Check sheet for the modelled part. Datum: model origin and axes. Units: mm. A direction names the side the tool comes from. Round coordinates to 2 decimals unless told otherwise and drop trailing zeros. Order: outer loops, then holes, each group sorted by start corner. A loop starts at its lowest first (then second) coordinate and runs counter-clockwise, first axis right, second up.
(1) Sectioned sample at A-A, the plane y = -25.5. Enter the section's corners in (x, z).
(2) Sectioned sample at C-C, the plane y = -32. Enter the section's corners in (x, z).
(3) Tool access check on faces 5 (the flat face through (-20, -45.939, -3)), 6 (the flat face through (18, -48, -11.938)), 7 (the flat face through (-19, -45, 20.828)), 8 (the flat face through (20, -46.99, -15)), 9 (the flat face through (0, -9, -16.51)). Record the directions out of +Z, -Z, +X, -X, +Y, -Y that give a thin tool (end or side, any length) a straight path to the whole face; none if there is none.
(4) Sectioned sample at B-B, the plane y = -40. Enter the section's corners in (x, z), and give its area (3 significant figures).
(5) Depth check by flat-ended pin: pin 1 (12.5 mm diameter, centred on x = -5.5, y = -47, fed in from -Z); pin 2 (16 mm diameter, centred on y = -41.5, z = -7.5, fed in from -X); pin 3 (1.5 mm diameter, centred on y = -15, z = 4, fed in from +X). Enter the tip coordinate at first touch or a pass-through.
(6) Mould release check, pull along Z, two halves, no side actions. Record for faces 1 (the flat face through (-18, -45, -22.86)), 2 (the cylindrical face through (-10.05, -4.29, 13.1)), 3 (the flat face through (14.195, -60.53, -0.107)), 4 (the flat face through (19, -45, -20.828)): released by +Z, released by -Z, zero draft, split by the parting line, or undercut.
(7) Thickness scan on probe 1 along Y at (x, z) = (19, 5.5); probe 2 along Z at (x, y) = (20.5, -54); probe 3 along Y at (x, z) = (6, -13). Record the ranges inside material, lowest first.
```python
from build123d import *

# Parameters (mm, degrees)
SKETCH1_R           = 12.446
BOSS_EXTRUDE1_DEPTH = 1.524
SKETCH2_R           = 16.51
BOSS_EXTRUDE2_DEPTH = 5.08
BOSS_EXTRUDE3_DEPTH = 5.842
FILLET1_R           = 0.508
FILLET2_R           = 0.508
SKETCH4_R           = 13.97
BOSS_EXTRUDE4_DEPTH = 4.064
BOSS_EXTRUDE5_DEPTH = 10.414
SKETCH6_W           = 22.86
SKETCH6_H           = 40.64
BOSS_EXTRUDE6_DEPTH = 34.798
SKETCH7_R           = 2.286
CUT_EXTRUDE1_DEPTH  = 9.398
SKETCH9_W           = 45.72
SKETCH9_H           = 34.798
BOSS_EXTRUDE7_DEPTH = 12.7
SKETCH10_W          = 41.656
SKETCH10_H          = 34.798
CUT_EXTRUDE2_DEPTH  = 9.652
CUT_EXTRUDE4_DEPTH  = 81.511990312
CUT_EXTRUDE5_DEPTH  = 81.511990312
SKETCH13_W          = 6.858
SKETCH13_H          = 1.524
BOSS_EXTRUDE8_DEPTH = 7.112
SKETCH14_W          = 6.604
SKETCH14_H          = 1.524
BOSS_EXTRUDE9_DEPTH = 7.112
SKETCH16_R          = 1.524
CUT_EXTRUDE7_DEPTH  = 7.112
SKETCH17_R          = 1.524
CUT_EXTRUDE8_DEPTH  = 12.7
FILLET3_R           = 1.27


with BuildPart() as part:
    # Sketch1 → Boss-Extrude1 (new body)
    with BuildSketch(Plane(origin=(0, 0, 0), x_dir=(1, 0, 0), z_dir=(0, 1, 0))):
        with Locations(Location((0, 0, 0), (0, 0, 270))):
            Circle(SKETCH1_R)
    extrude(amount=-BOSS_EXTRUDE1_DEPTH)

    # Sketch2 → Boss-Extrude2 (add)
    with BuildSketch(Plane.XZ.offset(1.524)):
        with Locations(Location((0, 0, 0), (0, 0, 270))):
            Circle(SKETCH2_R)
    extrude(amount=BOSS_EXTRUDE2_DEPTH)

    # Sketch3 → Boss-Extrude3 (add)
    with BuildSketch(Plane.XZ.offset(6.604)):
        Polygon((16.51, 7.366), (16.51, -7.366), (7.366, -16.51), (-7.366, -16.51), (-16.51, -7.366), (-16.51, 7.366), (-7.366, 16.51), (7.366, 16.51), align=None)
    extrude(amount=BOSS_EXTRUDE3_DEPTH)

    # Fillet1
    fillet1_edges = [part.edges().sort_by_distance(p)[0] for p in [
        (0, -1.524, 16.51),
    ]]
    fillet(fillet1_edges, radius=FILLET1_R)

    # Fillet2
    fillet2_edges = [part.edges().sort_by_distance(p)[0] for p in [
        (7.366, -9.525, -16.51),
        (16.51, -9.525, -7.366),
        (16.51, -9.525, 7.366),
        (7.366, -9.525, 16.51),
        (-7.366, -9.525, 16.51),
        (-16.51, -9.525, 7.366),
        (-16.51, -9.525, -7.366),
        (-7.366, -9.525, -16.51),
    ]]
    fillet(fillet2_edges, radius=FILLET2_R)

    # Sketch4 → Boss-Extrude4 (add)
    with BuildSketch(Plane.XZ.offset(12.446)):
        with Locations(Location((0, 0, 0), (0, 0, 270))):
            Circle(SKETCH4_R)
    extrude(amount=BOSS_EXTRUDE4_DEPTH)

    # Sketch5 → Boss-Extrude5 (add)
    with BuildSketch(Plane.XZ.offset(16.51)):
        with BuildLine():
            Line((12.7, 20.32), (-12.7, 20.32))
            ThreePointArc((-12.7, 20.32), (-18.088153673, 18.088153673), (-20.32, 12.7))
            Line((-20.32, 12.7), (-20.32, -12.7))
            ThreePointArc((-20.32, -12.7), (-18.088153673, -18.088153673), (-12.7, -20.32))
            Line((-12.7, -20.32), (12.7, -20.32))
            ThreePointArc((12.7, -20.32), (18.088153673, -18.088153673), (20.32, -12.7))
            Line((20.32, -12.7), (20.32, 12.7))
            ThreePointArc((20.32, 12.7), (18.088153673, 18.088153673), (12.7, 20.32))
        make_face()
    extrude(amount=BOSS_EXTRUDE5_DEPTH)

    # Sketch6 → Boss-Extrude6 (add)
    with BuildSketch(Plane.XZ.offset(26.924)):
        Rectangle(SKETCH6_W, SKETCH6_H)
    extrude(amount=BOSS_EXTRUDE6_DEPTH)

    # Sketch7 → Cut-Extrude1 (cut)
    with BuildSketch(Plane.XZ.offset(61.722)):
        with Locations(Location((0, -12.7, 0), (0, 0, 270))):
            Circle(SKETCH7_R)
        with Locations(Location((0, 12.7, 0), (0, 0, 270))):
            Circle(SKETCH7_R)
    extrude(amount=-CUT_EXTRUDE1_DEPTH, mode=Mode.SUBTRACT)

    # Sketch9 → Boss-Extrude7 (add)
    with BuildSketch(Plane(origin=(11.43, 0, 0), x_dir=(0, 0, -1), z_dir=(1, 0, 0))):
        with Locations((0, -44.323)):
            Rectangle(SKETCH9_W, SKETCH9_H)
    boss_extrude7 = extrude(amount=BOSS_EXTRUDE7_DEPTH)

    # Mirror1: Boss-Extrude7 across plane
    add(boss_extrude7.mirror(Plane(origin=(0, 0, 0), x_dir=(0, 0, 1), z_dir=(1, 0, 0))))

    # Sketch10 → Cut-Extrude2 (cut)
    with BuildSketch(Plane(origin=(24.13, 0, 0), x_dir=(0, 0, -1), z_dir=(1, 0, 0))):
        with Locations((0, -44.323)):
            Rectangle(SKETCH10_W, SKETCH10_H)
    cut_extrude2 = extrude(amount=-CUT_EXTRUDE2_DEPTH, mode=Mode.SUBTRACT)

    # Mirror2: Cut-Extrude2 across plane
    add(cut_extrude2.mirror(Plane(origin=(0, 0, 0), x_dir=(0, 0, 1), z_dir=(1, 0, 0))), mode=Mode.SUBTRACT)

    # Sketch11 → Cut-Extrude4 (cut, through all)
    with BuildSketch(Plane(origin=(0, 0, -22.86), x_dir=(-1, 0, 0), z_dir=(0, 0, -1))):
        Polygon((-11.43, -26.924), (-24.13, -32.874707767), (-24.13, -26.924), align=None)
        Polygon((24.13, -32.874707767), (24.13, -26.924), (11.43, -26.924), align=None)
        Polygon((11.326658159, -61.931639732), (24.061569251, -56.056015305), (24.026436821, -62.006619362), align=None)
        Polygon((-24.197589663, -55.77109271), (-24.232722094, -61.721696766), (-11.532943432, -61.796676397), align=None)
    extrude(amount=-CUT_EXTRUDE4_DEPTH, mode=Mode.SUBTRACT)

    # Sketch12 → Cut-Extrude5 (cut, through all)
    with BuildSketch(Plane(origin=(0, 0, -22.86), x_dir=(-1, 0, 0), z_dir=(0, 0, -1))):
        Polygon((27.344093716, -61.722), (27.344093716, -56.075395365), (24.061569251, -56.056015305), (20.546985538, -61.722), align=None)
    extrude(amount=-CUT_EXTRUDE5_DEPTH, mode=Mode.SUBTRACT)

    # Sketch13 → Boss-Extrude8 (add)
    with BuildSketch(Plane(origin=(14.478, 0, 0), x_dir=(0, 0, -1), z_dir=(1, 0, 0))):
        with Locations((-3.429, -47.752)):
            Rectangle(SKETCH13_W, SKETCH13_H)
        with Locations((15.367, -47.752)):
            Rectangle(SKETCH13_W, SKETCH13_H)
    extrude(amount=BOSS_EXTRUDE8_DEPTH)

    # Sketch14 → Boss-Extrude9 (add)
    with BuildSketch(Plane.ZY.offset(14.478)):
        with Locations((-3.302, -45.176922844)):
            Rectangle(SKETCH14_W, SKETCH14_H)
        with Locations((16.764, -45.176922844)):
            Rectangle(SKETCH14_W, SKETCH14_H)
    extrude(amount=BOSS_EXTRUDE9_DEPTH)

    # Sketch16 → Cut-Extrude7 (cut)
    with BuildSketch(Plane.XZ.offset(45.938922844)):
        with Locations(Location((-18.034, -3.302, 0), (0, 0, 270))):
            Circle(SKETCH16_R)
        with Locations(Location((-18.034, 16.764, 0), (0, 0, 270))):
            Circle(SKETCH16_R)
        with Locations((18.034, 3.429)):
            Circle(SKETCH16_R)
        with Locations((18.034, -15.367)):
            Circle(SKETCH16_R)
    extrude(amount=-CUT_EXTRUDE7_DEPTH, mode=Mode.SUBTRACT)

    # Sketch17 → Cut-Extrude8 (cut)
    with BuildSketch(Plane(origin=(0, -38.1, 0), x_dir=(1, 0, 0), z_dir=(0, 1, 0))):
        with Locations(Location((18.034, 15.367, 0), (0, 0, 270))):
            Circle(SKETCH17_R)
        with Locations(Location((18.034, -3.429, 0), (0, 0, 270))):
            Circle(SKETCH17_R)
    extrude(amount=-CUT_EXTRUDE8_DEPTH, mode=Mode.SUBTRACT)

    # Fillet3
    fillet3_edges = [part.edges().sort_by_distance(p)[0] for p in [
        (-11.43, -44.323, -22.86),
        (11.43, -44.323, -22.86),
        (-11.43, -44.323, 22.86),
        (11.43, -44.323, 22.86),
    ]]
    fillet(fillet3_edges, radius=FILLET3_R)


solid = part.part
```
Derived:
1. outline: (-20.32, -12.7) arc R7.62 ccw to (-12.7, -20.32) - (12.7, -20.32) arc R7.62 ccw to (20.32, -12.7) - (20.32, 12.7) arc R7.62 ccw to (12.7, 20.32) - (-12.7, 20.32) arc R7.62 ccw to (-20.32, 12.7) - close
2. outline: (-22.26, -22.86) - (-12.7, -22.86) arc R1.27 ccw to (-11.43, -21.59) - (-11.43, -20.32) - (11.43, -20.32) - (11.43, -21.59) arc R1.27 ccw to (12.7, -22.86) - (22.26, -22.86) - (22.26, -20.83) - (14.48, -20.83) - (14.48, 20.83) - (22.26, 20.83) - (22.26, 22.86) - (12.7, 22.86) arc R1.27 ccw to (11.43, 21.59) - (11.43, 20.32) - (-11.43, 20.32) - (-11.43, 21.59) arc R1.27 ccw to (-12.7, 22.86) - (-22.26, 22.86) - (-22.26, 20.83) - (-14.48, 20.83) - (-14.48, -20.83) - (-22.26, -20.83) - close
3. face 5: -X, -Y
3. face 6: +X, -Y
3. face 7: -X, +Y, -Y
3. face 8: +X
3. face 9: -Z, +X, -X, +Y
4. outline: (-24.13, -22.86) - (-12.7, -22.86) arc R1.27 ccw to (-11.43, -21.59) - (-11.43, -20.32) - (11.43, -20.32) - (11.43, -21.59) arc R1.27 ccw to (12.7, -22.86) - (24.13, -22.86) - (24.13, -20.83) - (14.48, -20.83) - (14.48, 20.83) - (24.13, 20.83) - (24.13, 22.86) - (12.7, 22.86) arc R1.27 ccw to (11.43, 21.59) - (11.43, 20.32) - (-11.43, 20.32) - (-11.43, 21.59) arc R1.27 ccw to (-12.7, 22.86) - (-24.13, 22.86) - (-24.13, 20.83) - (-14.48, 20.83) - (-14.48, -20.83) - (-24.13, -20.83) - close
4. area: 1,280 mm2
5. pin 1: stops at z = -22.43
5. pin 2: stops at x = -21.59
5. pin 3: stops at x = 13.59
6. face 1: released by -Z
6. face 2: split by the parting line
6. face 3: zero draft
6. face 4: undercut
7. probe 1: y = -48.51 to -46.99, -26.92 to -16.51
7. probe 2: z = -22.86 to -20.83, 20.83 to 22.86
7. probe 3: y = -61.72 to -16.51, -12.45 to -1.52
